from build123d import *


# Not quite as in the source:
# - a feature names something its author has since deleted; it is built from what else it names


with BuildPart() as f1:
    # F0 (on Front) → F1 (revolve)
    with BuildSketch(Plane.XZ):
        with BuildLine():
            ThreePointArc((-21.2629083544, 48.211786896), (-15.8463196743, 34.9304531122), (-14, 20.7063762118))
            Line((-14, 20.7063762118), (-14, 0))
            Line((-14, 0), (-12, 0))
            Line((-12, 0), (-12, 43))
            Line((-12, 43), (-7.5, 43))
            Line((-7.5, 43), (-7.5, 45))
            Line((-7.5, 45), (-15, 45))
            Line((-15, 45), (-21.5, 60.9745979309))
            Line((-21.5, 60.9745979309), (-21.5, 100))
            Line((-21.5, 100), (-31.5, 100))
            Line((-31.5, 100), (-27.405355799, 66.7795249261))
            ThreePointArc((-27.405355799, 66.7795249261), (-25.2508232926, 57.1924026226), (-21.2629083544, 48.211786896))
        make_face()
    revolve(axis=Axis((0, 0, -6.6078525846), (0, 0, -1)))


solid = f1.part
Geometry: final body of the model. Coordinates: model frame, mm. A direction names the side the tool comes from. Round coordinates to 2 decimals unless told otherwise and drop trailing zeros. Loops run counter-clockwise (first coordinate to the right, second up) from the corner with the lowest first, then second, coordinate; pieces in that order, holes last.
Q1. Access query for faces 1 (the flat face through (6, -5, 43)), 2 (the cylindrical face through (2.799, 21.317, 80.76)), 3 (the flat face through (21, -7, 100)). Directions: +Z, -Z, +X, -X, +Y, -Y. A direction counts if a zero-diameter tool reaches every point of the face in a straight line with its end or side. Return the directions, or none.
Q2. Section A-A on z = 31. Return loops of the section in (x, y).
Q3. Pin query (flat end, axial travel): P1, Ø12, axis at y = 4.5, z = 52.5, coming from the -X side; P2, Ø1, axis at x = -9.5, z = 75, coming from the -Y side; P3, Ø3, axis at x = -11, y = -21, coming from the -Z side. Return the tip coordinate at first contact, or that it passes through.
Q4. Pull-direction query (Y, two-part tool) for faces 4 (the flat face through (-4, 7, 45)), 5 (the flat face through (6.3, 10.4, 0)), 6 (the conical face through (22.989, -17.627, 79.466)); classes: released by +Y, released by -Y, zero draft, split by the parting line, or undercut.
Q5. Material intervals for L1, parallel to Y at x = 0, z = 9.5; L2, parallel to Y at x = 1, z = 67; L3, parallel to Z at x = 6.5, y = 10.5, sorted ascending.
Evaluation:
1. face 1: -Z
1. face 2: +Z
1. face 3: +Z, +X, -X, +Y, -Y
2. outline: circle Ø29.92 at (0, 0); hole circle Ø24 at (0, 0)
3. P1: stops at x = -25.44
3. P2: stops at y = -26.97
3. P3: stops at z = 49.95
4. face 4: undercut
4. face 5: zero draft
4. face 6: split by the parting line
5. L1: y = -14 to -12, 12 to 14
5. L2: y = -27.41 to -21.48, 21.48 to 27.41
5. L3: z = 0 to 45
